Geometry check sheet. Reference: drawing and pictorial views, mm from the part's lowest x, y, z. Give positions to 0.01 mm unless a question says otherwise; leave off trailing zeros. Write each loop counter-clockwise with the first axis right and the second up, starting at its lowest first coordinate (ties: lowest second). Pieces come first, ordered by that corner, then holes. Notation, with made-up numbers: M -6,43.25 L 28,43.25 A16 ccw 28,65.25 Z; hole C 15,-21.5 d7. An arc over 180 degrees is marked long. Answer as a JSON object with one key per item and string values.
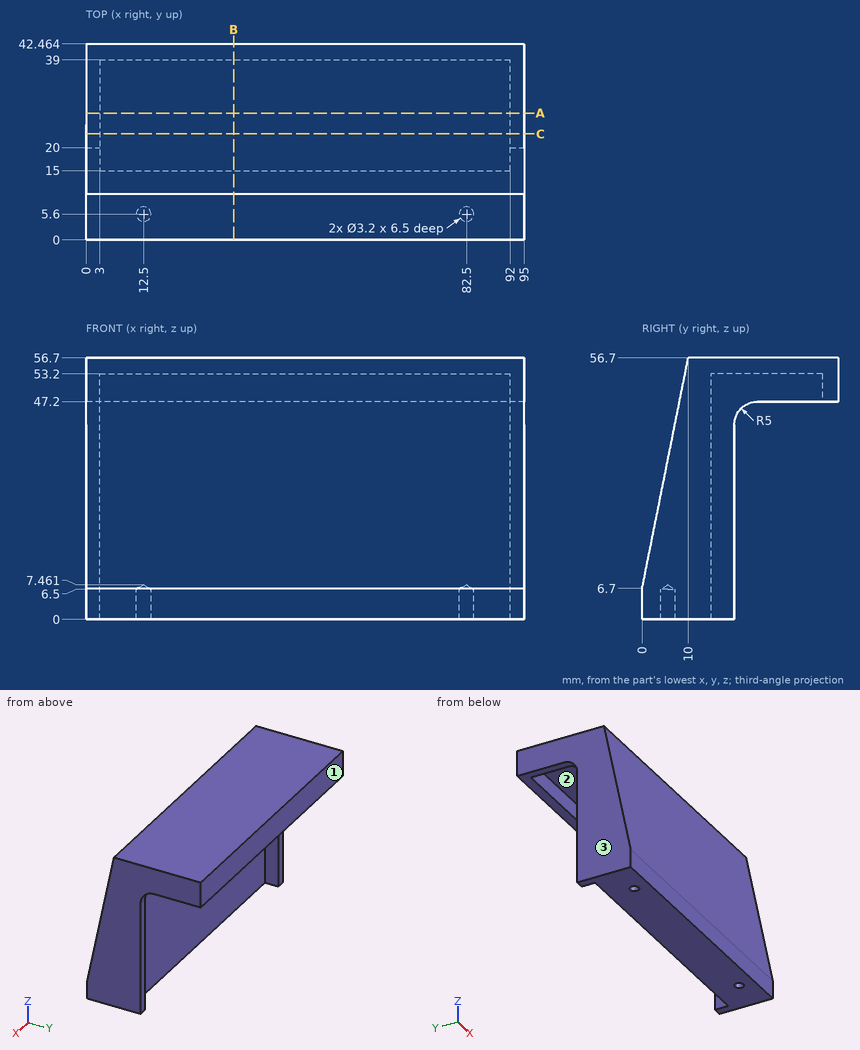
1) Go/stop test with flat-tipped pins: pin 1 (12 mm diameter, centred on x = 58.5, y = 23, fed in from -Z); pin 2 (10 mm diameter, centred on x = 54, z = 42.5, fed in from +Y); pin 3 (5 mm diameter, centred on x = 27, z = 49, fed in from -Y); pin 4 (8 mm diameter, centred on x = 44, z = 40.5, fed in from +Y). Record where each tip stops, or that it passes through.
Completed:
{"pin 1": "stops at z = 53.2", "pin 2": "stops at y = 42.46", "pin 3": "stops at y = 7.96", "pin 4": "stops at y = 15"}
2) Section check C-C on y = 23. Record the boundary of the cut face in (x, z).
Completed:
{"outline": "M 0,46.78 L 3,46.78 L 3,53.2 L 92,53.2 L 92,46.78 L 95,46.78 L 95,56.7 L 0,56.7 Z"}
3) Section check B-B on x = 32. Record the boundary of the cut face in (y, z).
Completed:
{"outline": "M 0,0 L 15,0 L 15,53.2 L 39,53.2 L 39,47.2 L 42.46,47.2 L 42.46,56.7 L 10,56.7 L 0,6.7 Z"}
4) Release check for a two-part mould opening along Y. For the marked faces 1, 2 and 3 record: pulls with the +Y half, pulls with the -Y half, needs draft (parallel to the pull), parting line crosses it, or undercut.
Completed:
{"face 1": "pulls with the +Y half", "face 2": "undercut", "face 3": "needs draft"}
5) Thickness scan on L1, parallel to Y at x = 82.5, z = 3.75; L2, parallel to X at y = 5, z = 5; L3, parallel to Z at x = 45.5, y = 20.5. Record the ranges inside material, lowest first.
Completed:
{"L1": "y = 0 to 4, 7.2 to 15", "L2": "x = 0 to 11.02, 13.98 to 81.02, 83.98 to 95", "L3": "z = 53.2 to 56.7"}
6) Section check A-A on y = 27.5. Record the boundary of the cut face in (x, z).
Completed:
{"outline": "M 0,47.2 L 3,47.2 L 3,53.2 L 92,53.2 L 92,47.2 L 95,47.2 L 95,56.7 L 0,56.7 Z"}
